Could you check a few things on this model? Use its own coordinates, in mm. A direction names the side the tool comes from. Round coordinates to 2 decimals unless told otherwise and drop trailing zeros. Write each loop counter-clockwise with the first axis right and the second up, starting at its lowest first coordinate (ties: lowest second). Pieces come first, ordered by that corner, then holes. Notation, with made-up numbers: (-31.75, 63.5) - (24.25, 63.5) arc R29 ccw to (24.25, 97.5) - close; hole circle Ø9 at (81, -7). An arc over 180 degrees is marked (long way). Write each question's results on one line, items separated by ' | '. Start each with the question number.
(1) On a 3-axis mill with a long thin cutter (end or side, diameter ignored), from which of +Z, -Z, +X, -X, +Y, -Y can I reach the whole of each face in a straight line? I mean faces 4 (the cylindrical face through (-19.37, 6.18, 10.19)), 5 (the flat face through (26, 1, 20.32)), 6 (the cylindrical face through (-47.5, -30.37, 3.13)), 7 (the cylindrical face through (-32.22, 6.18, 10.21)), 8 (the flat face through (-26, 6, 9.779)). Say none if no direction works.
(2) Imagine slicing it at B-B on x = -50.8. Write out the boundary of the cut face in (y, z).
(3) Please list where these lines run through material, in increasing order: line 1 (Y direction, x = -50.8, z = 6); line 2 (Y direction, x = -50.8, z = 6.75); line 3 (X direction, y = 1, z = 13.5). Write a range as [from, to].
(4) Imagine slicing it at A-A on x = 0. Write out the boundary of the cut face in (y, z), then the cut area to 3 significant figures.
(5) Imagine slicing it at D-D on z = 4.5. State how many separate pieces and enclosed holes the cut face has, then the cut area to 3 significant figures.
(6) Thinking about a two-plate mould opening in X: for faces 1 (the flat face through (-1, -3, 0)), 2 (the flat face through (-33.457, 6.18, 13.243)), 3 (the cylindrical face through (52.27, -4.38, 3.92)), which applies, +X half, -X half, draft (parallel to the pull), parting line (faces both ways), or undercut?
(7) Imagine slicing it at C-C on y = 5. Write out the boundary of the cut face in (x, z), then the cut area to 3 significant figures.
(8) For P1, Ø15.5, axis at x = -19, y = -16.5, coming from the +Z side; P2, Ø3.5, axis at x = 50.8, y = -30.226, coming from the -Z side; P3, Ø3, axis at x = 27, y = 5, coming from the -Z side; P4, Ø3, axis at y = 1.5, z = 15, coming from the -X side, each with a flat end and sliding along its axis, tell me the tip position at first contact or that it passes through.
```python
from build123d import *

# Parameters (mm, degrees)
SKETCH1_W          = 112.7252
SKETCH1_H          = 51.308
EXTRUDE1_DEPTH     = 1.6002
EXTRUDE2_REACH     = 78.632
SKETCH2_R          = 3.175
SKETCH2_R_2        = 3.302
SKETCH3_R          = 3.302
SKETCH3_R_2        = 1.4732
CUT_EXTRUDE1_DEPTH = 12.7
SKETCH4_W          = 31.242
SKETCH4_H          = 12.7
SKETCH4_W_2        = 39.4462
EXTRUDE3_DEPTH     = 3.556
EXTRUDE4_DEPTH     = 6.096


with BuildPart() as part:
    # Sketch1 → Extrude1 (new body)
    with BuildSketch(Plane.XY.offset(6.35)):
        with Locations((0, -25.654)):
            Rectangle(SKETCH1_W, SKETCH1_H)
    extrude(amount=EXTRUDE1_DEPTH)

    # Sketch2 → Extrude2 (add, up to next)
    with BuildSketch(Plane.XY, mode=Mode.PRIVATE) as extrude2_sk1:
        with Locations(Location((-50.8, -4.318, 0), (0, 0, 180))):
            Circle(SKETCH2_R)
    extrude2_tool1 = extrude(extrude2_sk1.sketch, amount=EXTRUDE2_REACH, mode=Mode.PRIVATE) - part.part
    # Sketch2 → Extrude2 (add, up to next)
    with BuildSketch(Plane.XY, mode=Mode.PRIVATE) as extrude2_sk2:
        with Locations(Location((50.8, -4.318, 0), (0, 0, 180))):
            Circle(SKETCH2_R)
    extrude2_tool2 = extrude(extrude2_sk2.sketch, amount=EXTRUDE2_REACH, mode=Mode.PRIVATE) - part.part
    # Sketch2 → Extrude2 (add, up to next)
    with BuildSketch(Plane.XY, mode=Mode.PRIVATE) as extrude2_sk3:
        with Locations(Location((-50.8, -30.226, 0), (0, 0, 180))):
            Circle(SKETCH2_R_2)
    extrude2_tool3 = extrude(extrude2_sk3.sketch, amount=EXTRUDE2_REACH, mode=Mode.PRIVATE) - part.part
    # Sketch2 → Extrude2 (add, up to next)
    with BuildSketch(Plane.XY, mode=Mode.PRIVATE) as extrude2_sk4:
        with Locations(Location((50.8, -30.226, 0), (0, 0, 180))):
            Circle(SKETCH2_R_2)
    extrude2_tool4 = extrude(extrude2_sk4.sketch, amount=EXTRUDE2_REACH, mode=Mode.PRIVATE) - part.part
    # Sketch2 → Extrude2 (add, up to next)
    with BuildSketch(Plane.XY, mode=Mode.PRIVATE) as extrude2_sk5:
        with Locations(Location((0, -4.318, 0), (0, 0, 180))):
            Circle(SKETCH2_R)
    extrude2_tool5 = extrude(extrude2_sk5.sketch, amount=EXTRUDE2_REACH, mode=Mode.PRIVATE) - part.part
    add(extrude2_tool1.solids().sort_by_distance((-50.8, -4.318, 0))[0])
    add(extrude2_tool2.solids().sort_by_distance((50.8, -4.318, 0))[0])
    add(extrude2_tool3.solids().sort_by_distance((-50.8, -30.226, 0))[0])
    add(extrude2_tool4.solids().sort_by_distance((50.8, -30.226, 0))[0])
    add(extrude2_tool5.solids().sort_by_distance((0, -4.318, 0))[0])

    # Sketch3 → Cut-Extrude1 (cut)
    with BuildSketch(Plane.XY):
        with Locations(Location((50.8, -42.418, 0), (0, 0, 180))):
            Circle(SKETCH3_R)
        with Locations(Location((0, -42.418, 0), (0, 0, 180))):
            Circle(SKETCH3_R)
        with Locations(Location((-50.8, -42.418, 0), (0, 0, 180))):
            Circle(SKETCH3_R)
        with Locations(Location((50.8, -30.226, 0), (0, 0, 180))):
            Circle(SKETCH3_R_2)
        with Locations(Location((50.8, -4.318, 0), (0, 0, 180))):
            Circle(SKETCH3_R_2)
        with Locations(Location((0, -4.318, 0), (0, 0, 180))):
            Circle(SKETCH3_R_2)
        with Locations(Location((-50.8, -4.318, 0), (0, 0, 180))):
            Circle(SKETCH3_R_2)
        with Locations(Location((-50.8, -30.226, 0), (0, 0, 180))):
            Circle(SKETCH3_R_2)
    extrude(amount=CUT_EXTRUDE1_DEPTH, mode=Mode.SUBTRACT)

    # Sketch4 → Extrude3 (add)
    with BuildSketch(Plane(origin=(0, 3.175, 0), x_dir=(-1, 0, 0), z_dir=(0, 1, 0))):
        with Locations((25.781, 13.97)):
            Rectangle(SKETCH4_W, SKETCH4_H)
        with Locations((-26.1493, 13.97)):
            Rectangle(SKETCH4_W_2, SKETCH4_H)
    extrude(amount=-EXTRUDE3_DEPTH)

    # Sketch5 → Extrude4 (add)
    with BuildSketch(Plane(origin=(0, 3.175, 0), x_dir=(1, 0, 0), z_dir=(0, 1, 0))):
        with BuildLine():
            Line((15.7353, -17.7038), (36.5633, -17.7038))
            ThreePointArc((36.5633, -17.7038), (38.175393987, -16.908803224), (38.526061279, -15.1458797))
            Line((38.526061279, -15.1458797), (37.491563037, -11.2850797))
            ThreePointArc((37.491563037, -11.2850797), (36.765804982, -10.198906013), (35.528801758, -9.779))
            Line((35.528801758, -9.779), (16.769798242, -9.779))
            ThreePointArc((16.769798242, -9.779), (15.532795018, -10.198906013), (14.807036963, -11.2850797))
            Line((14.807036963, -11.2850797), (13.772538721, -15.1458797))
            ThreePointArc((13.772538721, -15.1458797), (14.123206013, -16.908803224), (15.7353, -17.7038))
        make_face()
        with BuildLine():
            Line((-30.969501758, -9.779), (-20.592498242, -9.779))
            ThreePointArc((-20.592498242, -9.779), (-19.355495018, -10.198906013), (-18.629736963, -11.2850797))
            Line((-18.629736963, -11.2850797), (-17.595238721, -15.1458797))
            ThreePointArc((-17.595238721, -15.1458797), (-17.945906013, -16.908803224), (-19.558, -17.7038))
            Line((-19.558, -17.7038), (-32.004, -17.7038))
            ThreePointArc((-32.004, -17.7038), (-33.616093987, -16.908803224), (-33.966761279, -15.1458797))
            Line((-33.966761279, -15.1458797), (-32.932263037, -11.2850797))
            ThreePointArc((-32.932263037, -11.2850797), (-32.206504982, -10.198906013), (-30.969501758, -9.779))
        make_face()
    extrude(amount=EXTRUDE4_DEPTH)


solid = part.part
```
Response:
1) face 4: -Z, +Y | face 5: +Z, +X, -X, +Y, -Y | face 6: -Z | face 7: -Z, -X, +Y | face 8: -Z, +X, -X, +Y
2) outline: (-51.31, 6.35) - (-45.72, 6.35) - (-45.72, 7.95) - (-51.31, 7.95) - close; (-39.12, 6.35) - (-33.53, 6.35) - (-33.53, 0) - (-31.7, 0) - (-31.7, 7.95) - (-39.12, 7.95) - close; (-28.75, 0) - (-26.92, 0) - (-26.92, 6.35) - (-7.49, 6.35) - (-7.49, 0) - (-5.79, 0) - (-5.79, 7.95) - (-28.75, 7.95) - close; (-2.84, 0) - (-1.14, 0) - (-1.14, 6.35) - (0, 6.35) - (0, 7.95) - (-2.84, 7.95) - close
3) line 1: [-33.53, -31.7], [-28.75, -26.92], [-7.49, -5.79], [-2.84, -1.14] | line 2: [-51.31, -45.72], [-39.12, -31.7], [-28.75, -5.79], [-2.84, 0] | line 3: [-41.4, -10.16], [6.43, 45.87]
4) outline: (-51.31, 6.35) - (-45.72, 6.35) - (-45.72, 7.95) - (-51.31, 7.95) - close; (-39.12, 6.35) - (-7.49, 6.35) - (-7.49, 0) - (-5.79, 0) - (-5.79, 7.95) - (-39.12, 7.95) - close; (-2.84, 0) - (-1.14, 0) - (-1.14, 6.35) - (0, 6.35) - (0, 7.95) - (-2.84, 7.95) - close | area: 88.4 mm²
5) separate pieces: 5 | enclosed holes: 5 | area: 129 mm²
6) face 1: draft | face 2: -X half | face 3: undercut
7) outline: (-33.97, 15.15) - (-32.93, 11.29) arc R2.03 ccw to (-30.97, 9.78) - (-20.59, 9.78) arc R2.03 ccw to (-18.63, 11.29) - (-17.6, 15.15) arc R2.03 ccw to (-19.56, 17.7) - (-32, 17.7) arc R2.03 ccw to start; (13.77, 15.15) - (14.81, 11.29) arc R2.03 ccw to (16.77, 9.78) - (35.53, 9.78) arc R2.03 ccw to (37.49, 11.29) - (38.53, 15.15) arc R2.03 ccw to (36.56, 17.7) - (15.74, 17.7) arc R2.03 ccw to start | area: 306 mm²
8) P1: z = 7.95 | P2: z = 0 | P3: z = 9.78 | P4: x = -41.4
